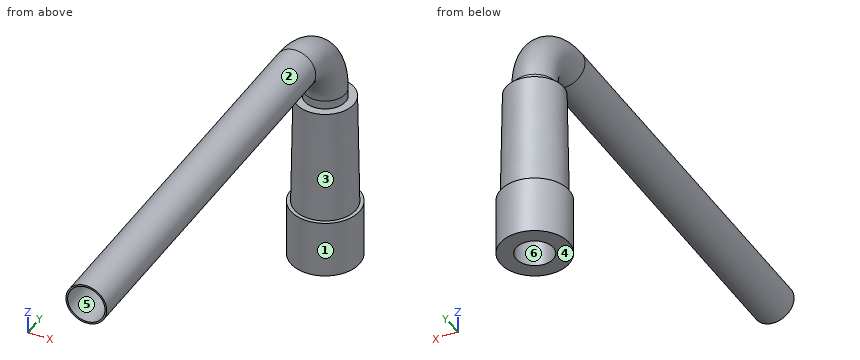
Autodesk Inventor part; units mm, degrees
ref_plane "YZ Plane" through (0, 0, 0) normal (1, 0, 0) x (0, 1, 0)
ref_plane "XZ Plane" through (0, 0, 0) normal (0, 1, 0) x (-1, 0, 0)
ref_plane "XY Plane" through (0, 0, 0) normal (0, 0, 1) x (1, 0, 0)
sketch "Esboço1" plane through (0, 0, 0) normal (0, 0, 1) x (1, 0, 0)
  circle A0 centre (0, 0) radius 3.25
  circle A1 centre (0, 0) radius 6
  point P0 (0, 0)
  dimension "d0" = 12
extrude "Extrusão1" add sketch "Esboço1" along normal mid plane 10
sketch "Esboço2" plane through (0, 0, 5) normal (0, 0, 1) x (1, 0, 0)
  circle A0 centre (0, 0) radius 6
  circle A1 centre (0, 0) radius 5
  circle A2 centre (0, 0) radius 3.25
  point P0 (0, 0)
  dimension "d3" = 1
extrude "Extrusão2" add sketch "Esboço2" along normal blind 20 contours A1
draft "Face para inclinação de faces1" angle 1 pull direction (0, 0, 1) faces at (4.9353, -0.8021, 18.3333) fixed edges at (-5, 0, 25)
sketch "Esboço3" plane through (0, 0, 25) normal (0, 0, 1) x (1, 0, 0)
  circle A0 centre (0, 0) radius 3.25
  circle A1 centre (0, 0) radius 3.55
  point P0 (0, 0)
  dimension "d7" = 0.3
sketch3d "Esboço 3D1"
  line L0 (0, 0, 25) -> (0, 0, 26.4983)
  arc A0 (0, 0, 26.4983) -> (0, -10, 36.4983) centre (0, -10, 26.4983) ccw
  line L1 (0, -10, 36.4983) -> (0, -80, 36.4983)
  dimension "d8" = 80
  dimension "d9" = 10
sweep "Varredura1" add profiles "Esboço3" path "Esboço 3D1"
properties part number "Tubo de Entrada do Ar"
Build history of the part. All positions in model axes, mm. Face numbers are marked on the shaded views. A direction names the side the tool comes from. Round coordinates to 2 decimals unless told otherwise and drop trailing zeros. Write each loop counter-clockwise with the first axis right and the second up, starting at its lowest first coordinate (ties: lowest second). Pieces come first, ordered by that corner, then holes. Notation, with made-up numbers: (-22.5, -14.5) - (24.5, -14.5) arc R22 ccw to (24.5, 14.5) - close; hole circle Ø2 at (35.25, 53). An arc over 180 degrees is marked (long way). One line per question, with ' | ' between items.
1. Mould opens along X. For the marked faces 3, 4, 5 and 6 say: released by +X, released by -X, zero draft, split by the parting line, or undercut.
Results are:
face 3: split by the parting line | face 4: zero draft | face 5: undercut | face 6: undercut
2. Drop flat-ended pins along their axis: pin 1 Ø6 at (x, z) = (3.5, 6) entering from -Y; pin 2 Ø5 at (x, y) = (-1, -25) entering from +Z; pin 3 Ø5 at (x, y) = (-0.5, -0.5) entering from +Z; pin 4 Ø1.5 at (x, y) = (0, -46.5) entering from -Z. Give the stop position or say it passes through.
Results are:
pin 1: y = -5.96 | pin 2: z = 40.05 | pin 3: z = 38.08 | pin 4: z = 32.95
3. Band-saw the part on A-A, the plane z = 17.5. Write the cut outline in (x, y).
Results are:
outline: circle Ø10.26 at (0, 0); hole circle Ø6.5 at (0, 0)
4. Band-saw the part on B-B, the plane y = -41.5. Write the cut outline in (x, z), and give its area (3 significant figures).
Results are:
outline: circle Ø7.1 at (0, 36.5); hole circle Ø6.5 at (0, 36.5) | area: 6.41 mm^2
5. Drill centre lines: line 1 along Z through (x, y) = (-0.25, -16.5); line 2 along Z through (x, y) = (0, -64.5); line 3 along Y through (x, z) = (-1.75, 10.5). Where is each one in solid material? Low to high. Write a range as from..to.
Results are:
line 1: 32.96..33.26, 39.74..40.04 | line 2: 32.95..33.25, 39.75..40.05 | line 3: -4.95..-2.74, 2.74..4.95
6. Tool access for the marked faces 1 and 2: list every direction of +Z, -Z, +X, -X, +Y, -Y with a clear straight run to the whole face (end or side of a thin tool).
Results are:
face 1: -Z | face 2: -Y
